For this review, take the finished solid that the model builds, in its own axes (mm). A direction names the side the tool comes from. Give positions to 0.01 mm unless a question says otherwise; leave off trailing zeros. Loops run counter-clockwise (first coordinate to the right, second up) from the corner with the lowest first, then second, coordinate; pieces in that order, holes last. Notation, with made-up numbers: (69, 64.5) - (96, 64.5) arc R18 cw to (96, 74.5) - close; hole circle Ø11 at (52, 62). An arc over 180 degrees is marked (long way). Put each result on its own line as item: value.
Autodesk Inventor part; units mm, degrees
ref_plane "YZ Plane" through (0, 0, 0) normal (1, 0, 0) x (0, 1, 0)
ref_plane "XZ Plane" through (0, 0, 0) normal (0, 1, 0) x (-1, 0, 0)
ref_plane "XY Plane" through (0, 0, 0) normal (0, 0, 1) x (1, 0, 0)
sketch "スケッチ1" plane through (0, 0, 0) normal (0, 0, 1) x (1, 0, 0)
  circle A0 centre (0, 0) radius 2.5
  dimension "d0" = 5
extrude "押し出し1" add sketch "スケッチ1" along normal blind 32
sketch "スケッチ2" plane through (0, 0, 32) normal (0, 0, 1) x (1, 0, 0)
  circle A0 centre (0, 0) radius 2
  dimension "d3" = 4
extrude "押し出し2" cut sketch "スケッチ2" against normal blind 6
thread "ねじ1"
chamfer "面取り1" distance 0.05 angle 45 2 edges at (-2.5, 0, 32) (-2.5, 0, 0)
properties part number "shaft_31.6mm_Φ5" material "アルミニウム 7075"
1) For faces 4 (the face through (0, 0, 0)), 5 (the face through (0, -2, 29)), list the 3-axis set-ups (+Z, -Z, +X, -X, +Y, -Y) from which the entire face can be reached by the end or side of a thin tool; tool diameter is ignored.
Geometry check:
face 4: -Z, +X, -X, +Y, -Y
face 5: +Z
2) Insertion check: pin 1 Ø2.5 at (x, y) = (0, 0) entering from +Z; pin 2 Ø2 at (y, z) = (1.5, 15.5) entering from +X. Each pin has a flat end and moves straight along its axis. Give the tip position at first contact, or say it passes through.
Geometry check:
pin 1: stops at z = 26
pin 2: stops at x = 2.45
3) Wall thickness on line 1 (Y direction, x = 0, z = 30.6); line 2 (Z direction, x = 1.65, y = 0); line 3 (X direction, y = -1.75, z = 19.5): over which ranges is each line inside the solid? List them lowest first.
Geometry check:
line 1: y = -2.5 to -2, 2 to 2.5
line 2: z = 0 to 26
line 3: x = -1.79 to 1.79
4) Draft analysis for pull direction X (two halves, no side actions). For faces 1 (the face through (0, 0, 26)), 2 (the face through (-0.54, 2.44, 15.78)), 3 (the face through (-1, -2, 32)), state which applies: pulls with the +X half, pulls with the -X half, needs draft (parallel to the pull), parting line crosses it, or undercut.
Geometry check:
face 1: undercut
face 2: parting line crosses it
face 3: needs draft
5) Take a section at D-D on z = 11. State the section outline as (x, y) points, and give its area (3 significant figures).
Geometry check:
outline: circle Ø5 at (0, 0)
area: 19.6 mm²
6) Take a section at A-A on y = 0. State the section outline as (x, z) points, and give its area (3 significant figures).
Geometry check:
outline: (-2.5, 0.05) - (-2.45, 0) - (2.45, 0) - (2.5, 0.05) - (2.5, 31.95) - (2.45, 32) - (2, 32) - (2, 26) - (-2, 26) - (-2, 32) - (-2.45, 32) - (-2.5, 31.95) - close
area: 136 mm²
7) Take a section at B-B on z = 29. State the section outline as (x, y) points, and give its area (3 significant figures).
Geometry check:
outline: circle Ø5 at (0, 0); hole circle Ø4 at (0, 0)
area: 7.07 mm²
